The model under review builds one solid part; all positions refer to its coordinate system, in mm. A direction names the side the tool comes from. Coordinates: 2 decimals unless noted, no trailing zeros. Loops run counter-clockwise (first coordinate to the right, second up) from the corner with the lowest first, then second, coordinate; pieces in that order, holes last. Notation, with made-up numbers: M 75.5,23.5 L 108.5,23.5 A35 cw 108.5,62.5 Z; hole C -2,-18.75 d8. An arc over 180 degrees is marked long. Use one line per item in the form item = value.
```python
from build123d import *

# Parameters (mm, degrees)
F1_DEPTH = 30
F3_D     = 3
F5_D     = 9
F5_DEPTH = 4
F5_TIP   = 2.7038727856
F7_D     = 3
F9_D     = 8
F9_DEPTH = 4
F9_TIP   = 2.4034424761


with BuildPart() as f1:
    # F0 (on Top) → F1 (new body)
    with BuildSketch(Plane.XY):
        with BuildLine():
            ThreePointArc((-0.3734174669, 52.9050653557), (-0.1966407716, 52.831842051), (-0.1234174669, 52.6550653557))
            Line((-0.1234174669, 52.6550653557), (-0.1234174669, 9.9050653557))
            ThreePointArc((-0.1234174669, 9.9050653557), (-1.5878835609, 6.3695314498), (-5.1234174669, 4.9050653557))
            Line((-5.1234174669, 4.9050653557), (-40.1234174669, 4.9050653557))
            Line((-40.1234174669, 4.9050653557), (-40.1234174669, 0.9050653557))
            Line((-40.1234174669, 0.9050653557), (-1.1234174669, 0.9050653557))
            ThreePointArc((-1.1234174669, 0.9050653557), (2.4121164391, 2.3695314498), (3.8765825331, 5.9050653557))
            Line((3.8765825331, 5.9050653557), (3.8765825331, 53.9050653557))
            ThreePointArc((3.8765825331, 53.9050653557), (2.4121164391, 57.4405992616), (-1.1234174669, 58.9050653557))
            Line((-1.1234174669, 58.9050653557), (-40.1234174669, 58.9050653557))
            Line((-40.1234174669, 58.9050653557), (-40.1234174669, 52.9050653557))
            Line((-40.1234174669, 52.9050653557), (-0.3734174669, 52.9050653557))
        make_face()
    extrude(amount=F1_DEPTH)

    # F3 (through all)
    with Locations(Plane.YZ.offset(3.8765825331)):
        with Locations((23.0537810803, 17.4629910993), (27.4050653557, 10), (31.7563496311, 17.4629910993)):
            Hole(F3_D / 2)

    # F5
    with Locations(Plane(origin=(0, 58.9050653557, 0), x_dir=(-1, 0, 0), z_dir=(0, 1, 0))):
        with Locations((24.1229310632, 15)):
            Hole(F5_D / 2, depth=F5_DEPTH)
            with Locations((0, 0, -(F5_DEPTH + F5_TIP / 2))):  # 118° drill point
                Cone(0, F5_D / 2, F5_TIP, mode=Mode.SUBTRACT)

    # F7 (through all)
    with Locations(Plane(origin=(0, 58.9050653557, 0), x_dir=(-1, 0, 0), z_dir=(0, 1, 0))):
        with Locations((31.6229310632, 15), (24.1229310632, 7.5), (16.8729310632, 15)):
            Hole(F7_D / 2)

    # F9
    with Locations(Plane.XZ.offset(-0.9050653557)):
        with Locations((-24.1234174669, 15)):
            Hole(F9_D / 2, depth=F9_DEPTH)
            with Locations((0, 0, -(F9_DEPTH + F9_TIP / 2))):  # 118° drill point
                Cone(0, F9_D / 2, F9_TIP, mode=Mode.SUBTRACT)


solid = f1.part
```
1. Add section A-A (x = -9). State the section outline as (y, z) points.
Response values:
outline = M 0.91,0 L 4.91,0 L 4.91,30 L 0.91,30 Z; M 52.91,0 L 58.91,0 L 58.91,30 L 52.91,30 Z
2. Insertion check: P1, Ø7, axis at x = -24.12, z = 15, coming from the +Y side; P2, Ø6, axis at y = 40, z = 13.5, coming from the -X side. Each pin has a flat end and moves straight along its axis. Give the tip position at first contact, or say it passes through.
Response values:
P1 = 54.31
P2 = -0.12
3. The part is to be moulded in two halves that separate along Y. For faces 1 (the face through (2.45, 57.4, 14.79)), 2 (the face through (1.85, 32.86, 18.48)), 3 (the face through (3.877, 30, 15)), say which applies: pulls with the +Y half, pulls with the -Y half, needs draft (parallel to the pull), parting line crosses it, or undercut.
Response values:
face_1 = pulls with the +Y half
face_2 = undercut
face_3 = needs draft
4. Add section D-D (y = 42.5). State the section outline as (x, z) points.
Response values:
outline = M -0.12,0 L 3.88,0 L 3.88,30 L -0.12,30 Z
5. Add section B-B (z = 24.75). State the section outline as (x, y) points.
Response values:
outline = M -40.12,0.91 L -1.12,0.91 A5 ccw 3.88,5.91 L 3.88,53.91 A5 ccw -1.12,58.91 L -40.12,58.91 L -40.12,52.91 L -0.37,52.91 A0.25 cw -0.12,52.66 L -0.12,9.91 A5 cw -5.12,4.91 L -40.12,4.91 Z
6. Add section C-C (z = 7.5). State the section outline as (x, y) points.
Response values:
outline = M -40.12,0.91 L -25.62,0.91 L -25.62,4.91 L -40.12,4.91 Z; M -40.12,52.91 L -25.62,52.91 L -25.62,58.91 L -40.12,58.91 Z; M -22.62,0.91 L -1.12,0.91 A5 ccw 3.88,5.91 L 3.88,53.91 A5 ccw -1.12,58.91 L -22.62,58.91 L -22.62,52.91 L -0.37,52.91 A0.25 cw -0.12,52.66 L -0.12,9.91 A5 cw -5.12,4.91 L -22.62,4.91 Z
7. Machinability: for faces 4 (the face through (-20.127, 2.933, 15.176)), 5 (the face through (-23.43, 2.88, 6.17)), 6 (the face through (-0.123, 32, 15)), which of the approach directions +Z, -Z, +X, -X, +Y, -Y give a long, thin tool a straight path to every point of the face, cutting with its end or side? Answer none if there is none.
Response values:
face_4 = -Y
face_5 = +Y, -Y
face_6 = +Z, -Z, -X
8. Wall thickness on line 1 along Y through (x, z) = (-35, 25.25); line 2 along Y through (x, z) = (-2, 13.75); line 3 along X through (y, z) = (25, 3.25): over which ranges is each line inside the solid? List them lowest first. Write a range as from..to.
Response values:
line_1 = 0.91..4.91, 52.91..58.91
line_2 = 0.91..6, 52.91..58.91
line_3 = -0.12..3.88
